Part print with two shaded views. Sizes in mm from the minimum x, y, z corner. A direction names the side the tool comes from. Round coordinates to 2 decimals unless told otherwise and drop trailing zeros. Loops run counter-clockwise (first coordinate to the right, second up) from the corner with the lowest first, then second, coordinate; pieces in that order, holes last. Notation, with made-up numbers: M 67,56.5 L 116,56.5 A26 ccw 116,75.5 Z; hole C 11,-23 d6. An arc over 180 degrees is marked long. Put each result on its own line as item: value. Start each with the question number.
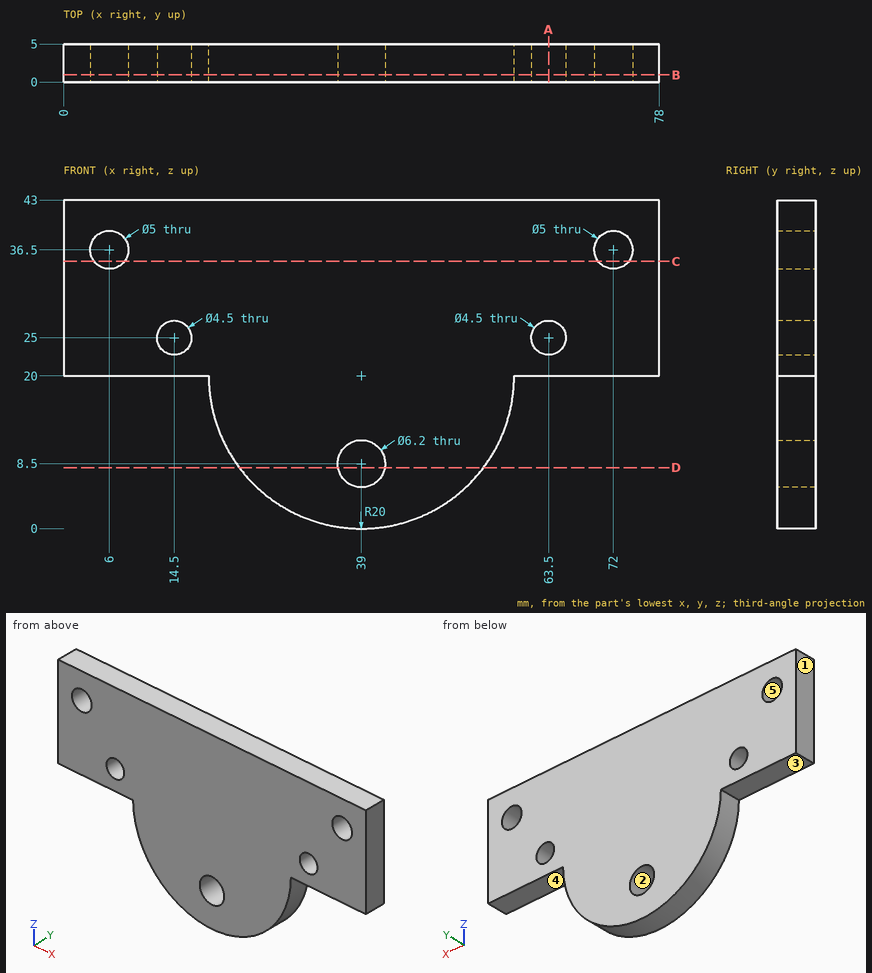
(1) Cut at A-A on x = 63.5. List the corners of the cut face in (y, z), and give its area (3 significant figures).
(2) Mould opens along X. For the marked faces 1, 2 and 3 say: +X half, -X half, draft (parallel to the pull), parting line (faces both ways), or undercut.
(3) Tool access for the marked faces 4 and 5: list every direction of +Z, -Z, +X, -X, +Y, -Y with a clear straight run to the whole face (end or side of a thin tool).
(4) Drill centre lines: line 1 along X through (y, z) = (1.65, 25); line 2 along X through (y, z) = (3.25, 36.5); line 3 along Z through (x, y) = (72, 2.45). Where is each one in solid material? Low to high.
(5) Cut at C-C on z = 35. List the corners of the cut face in (x, y), and give its area (3 significant figures).
(6) Cut at D-D on z = 8. List the corners of the cut face in (x, y), and give its area (3 significant figures).
(7) Cut at B-B on y = 0.95. List the corners of the cut face in (x, z), and give its area (3 significant figures).
Taken from the geometry:
1. outline: M 0,20 L 5,20 L 5,22.75 L 0,22.75 Z; M 0,27.25 L 5,27.25 L 5,43 L 0,43 Z
1. area: 92.5 mm2
2. face 1: -X half
2. face 2: undercut
2. face 3: draft
3. face 4: -Z, +X, +Y, -Y
3. face 5: +Y, -Y
4. line 1: 0 to 12.25, 16.75 to 61.25, 65.75 to 78
4. line 2: 0 to 3.5, 8.5 to 69.5, 74.5 to 78
4. line 3: 20 to 34, 39 to 43
5. outline: M 0,0 L 4,0 L 4,5 L 0,5 Z; M 8,0 L 70,0 L 70,5 L 8,5 Z; M 74,0 L 78,0 L 78,5 L 74,5 Z
5. area: 350 mm2
6. outline: M 23,0 L 35.94,0 L 35.94,5 L 23,5 Z; M 42.06,0 L 55,0 L 55,5 L 42.06,5 Z
6. area: 129 mm2
7. outline: M 0,20 L 19,20 A20 ccw 59,20 L 78,20 L 78,43 L 0,43 Z; hole C 6,36.5 d5; hole C 14.5,25 d4.5; hole C 39,8.5 d6.2; hole C 63.5,25 d4.5; hole C 72,36.5 d5
7. area: 2,320 mm2
